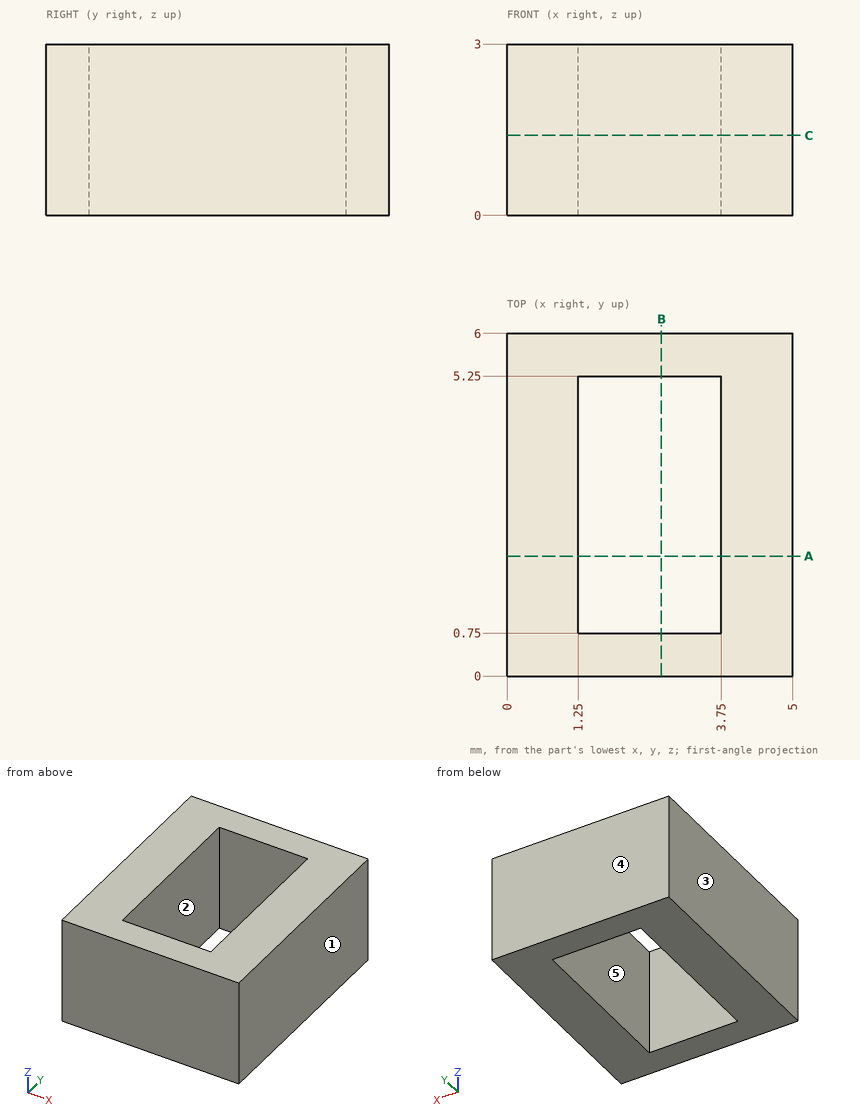
Geometry: see drawing. Coordinates: mm, zero at the bounding-box minimum. A direction names the side the tool comes from. Give positions to 0.01 mm unless a question says otherwise; leave off trailing zeros. Order: outer loops, then holes, each group sorted by start corner. A loop starts at its lowest first (then second) coordinate and runs counter-clockwise, first axis right, second up.
1. Cut plane A-A (y = 2.1). Return loops of the section in (x, z), and give its area (3 significant figures).
Computed:
outline: (0, 0) - (1.25, 0) - (1.25, 3) - (0, 3) - close; (3.75, 0) - (5, 0) - (5, 3) - (3.75, 3) - close
area: 7.50 mm2
2. Draft query along X for the marked faces 1, 2 and 3. Return one class per face: released by +X, released by -X, zero draft, split by the parting line, or undercut.
Computed:
face 1: released by +X
face 2: undercut
face 3: released by -X
3. Set-up query: the marked faces 4 and 5. Return all of +Z, -Z, +X, -X, +Y, -Y with unobstructed straight access to the full face (end or side cutting, diameter ignored); none if empty.
Computed:
face 4: +Z, -Z, +X, -X, +Y
face 5: +Z, -Z
4. Line query: probe 1 along X at (y, z) = (1.8, 2.9); probe 2 along Y at (x, z) = (1.3, 2.4). Output: solid intervals per line, ascending.
Computed:
probe 1: x = 0 to 1.25, 3.75 to 5
probe 2: y = 0 to 0.75, 5.25 to 6
5. Cut plane C-C (z = 1.4). Return loops of the section in (x, y), and give its area (4 significant figures).
Computed:
outline: (0, 0) - (5, 0) - (5, 6) - (0, 6) - close; hole (1.25, 0.75) - (3.75, 0.75) - (3.75, 5.25) - (1.25, 5.25) - close
area: 18.75 mm2
6. Cut plane B-B (x = 2.7). Return loops of the section in (y, z).
Computed:
outline: (0, 0) - (0.75, 0) - (0.75, 3) - (0, 3) - close; (5.25, 0) - (6, 0) - (6, 3) - (5.25, 3) - close
